```python
from build123d import *

# Parameters (mm, degrees)
ESQUISSE1_W                   = 44.2
ESQUISSE1_H                   = 52.2
BOSS_EXTRU_1_DEPTH            = 52.2
ENL_V_MAT_EXTRU_2_DEPTH       = 74.209903702
ENL_V_MAT_EXTRU_2_DEPTH_BACK  = 44.2
ENL_V_MAT_EXTRU_3_DEPTH       = 74.209903702
ENL_V_MAT_EXTRU_3_DEPTH_BACK  = 44.2
ENL_V_MAT_EXTRU_4_DEPTH       = 78.059003368
ENL_V_MAT_EXTRU_4_DEPTH_BACK  = 46
ENL_V_MAT_EXTRU_5_DEPTH       = 78.059003368
ENL_V_MAT_EXTRU_5_DEPTH_BACK  = 46
ENL_V_MAT_EXTRU_7_DEPTH       = 45.550224466
ENL_V_MAT_EXTRU_7_DEPTH_BACK  = 45.550224466
ENL_V_MAT_EXTRU_8_DEPTH       = 78.059003368
ENL_V_MAT_EXTRU_8_DEPTH_BACK  = 46
ENL_V_MAT_EXTRU_9_DEPTH       = 75.993733072
ENL_V_MAT_EXTRU_9_DEPTH_BACK  = 46
ESQUISSE13_W                  = 35
ESQUISSE13_H                  = 43
ENL_V_MAT_EXTRU_10_DEPTH      = 44
ENL_V_MAT_EXTRU_11_DEPTH      = 72.032809321
ENL_V_MAT_EXTRU_11_DEPTH_BACK = 1.5
ENL_V_MAT_EXTRU_13_DEPTH      = 72.032809321
ENL_V_MAT_EXTRU_13_DEPTH_BACK = 38
ENL_V_MAT_EXTRU_15_DEPTH      = 71.818217995
ENL_V_MAT_EXTRU_15_DEPTH_BACK = 46


with BuildPart() as part:
    # Esquisse1 → Boss.-Extru.1 (new body)
    with BuildSketch(Plane.XY):
        Rectangle(ESQUISSE1_W, ESQUISSE1_H)
    extrude(amount=BOSS_EXTRU_1_DEPTH)

    # Esquisse2 → Enlèv. mat.-Extru.2 (cut, two sides: drawn at the far end of the back side and taken through both)
    with BuildSketch(Plane(origin=(22.1, 0, 0), x_dir=(0, 0, -1), z_dir=(1, 0, 0)).offset(-ENL_V_MAT_EXTRU_2_DEPTH_BACK)):
        Polygon((-201.352290675, -19.9), (-52.2, -19.9), (-28.55, -19.9), (-28.55, -21.45), (-32.25, -21.45), (-32.25, -22.45), (-28.745559959, -26.1), (74.553898465, -133.690091099), (-39.180744024, -409.461834307), (-315.086933163, -295.671743208), align=None)
    extrude(amount=ENL_V_MAT_EXTRU_2_DEPTH + ENL_V_MAT_EXTRU_2_DEPTH_BACK, mode=Mode.SUBTRACT)

    # Esquisse3 → Enlèv. mat.-Extru.3 (cut, two sides: drawn at the far end of the back side and taken through both)
    with BuildSketch(Plane(origin=(22.1, 0, 0), x_dir=(0, 0, -1), z_dir=(1, 0, 0)).offset(-ENL_V_MAT_EXTRU_3_DEPTH_BACK)):
        Polygon((149.152290675, -19.9), (0, -19.9), (-23.65, -19.9), (-23.65, -21.45), (-19.95, -21.45), (-19.95, -22.45), (-23.454440041, -26.1), (-126.753898465, -133.690091099), (-13.019255976, -409.461834307), (262.886933163, -295.671743208), align=None)
    extrude(amount=ENL_V_MAT_EXTRU_3_DEPTH + ENL_V_MAT_EXTRU_3_DEPTH_BACK, mode=Mode.SUBTRACT)

    # Esquisse4 → Enlèv. mat.-Extru.4 (cut, two sides: drawn at the far end of the back side and taken through both)
    with BuildSketch(Plane(origin=(0, 26.1, 0), x_dir=(1, 0, 0), z_dir=(0, 1, 0)).offset(-ENL_V_MAT_EXTRU_4_DEPTH_BACK)):
        Polygon((-15.9, -191.333109619), (-15.9, -52.2), (-15.9, -28.55), (-17.45, -28.55), (-17.45, -32.25), (-18.45, -32.25), (-22.1, -28.745559959), (-122.462816227, 67.614843274), (-379.791464965, -38.281593439), (-273.228648738, -297.229546332), align=None)
    extrude(amount=ENL_V_MAT_EXTRU_4_DEPTH + ENL_V_MAT_EXTRU_4_DEPTH_BACK, mode=Mode.SUBTRACT)

    # Esquisse5 → Enlèv. mat.-Extru.5 (cut, two sides: drawn at the far end of the back side and taken through both)
    with BuildSketch(Plane(origin=(0, 26.1, 0), x_dir=(1, 0, 0), z_dir=(0, 1, 0)).offset(-ENL_V_MAT_EXTRU_5_DEPTH_BACK)):
        Polygon((-15.9, 139.133109619), (-15.9, 0), (-15.9, -23.65), (-17.45, -23.65), (-17.45, -19.95), (-18.45, -19.95), (-22.1, -23.454440041), (-122.462816228, -119.814843274), (-379.791464965, -13.918406561), (-273.228648738, 245.029546332), align=None)
    extrude(amount=ENL_V_MAT_EXTRU_5_DEPTH + ENL_V_MAT_EXTRU_5_DEPTH_BACK, mode=Mode.SUBTRACT)

    # Esquisse6 → Enlèv. mat.-Extru.7 (cut, two sides: drawn at the far end of the back side and taken through both)
    with BuildSketch(Plane.XY.offset(28.55).offset(-ENL_V_MAT_EXTRU_7_DEPTH_BACK)):
        Polygon((-161.22284167, -19.9), (-22.1, -19.9), (-15.9, -19.9), (-15.9, -26.093649616), (-15.9, -165.216491285), (-212.645110561, -361.97019968), (-357.967952231, -216.653708395), align=None)
    extrude(amount=ENL_V_MAT_EXTRU_7_DEPTH + ENL_V_MAT_EXTRU_7_DEPTH_BACK, mode=Mode.SUBTRACT)

    # Esquisse11 → Enlèv. mat.-Extru.8 (cut, two sides: drawn at the far end of the back side and taken through both)
    with BuildSketch(Plane(origin=(0, 26.1, 0), x_dir=(1, 0, 0), z_dir=(0, 1, 0)).offset(-ENL_V_MAT_EXTRU_8_DEPTH_BACK)):
        Polygon((164.227968273, -49.1), (22.1, -49.1), (-15.9, -49.1), (-158.027968273, -49.1), (-158.027968273, -333.355936546), (164.227968273, -333.355936546), align=None)
    extrude(amount=ENL_V_MAT_EXTRU_8_DEPTH + ENL_V_MAT_EXTRU_8_DEPTH_BACK, mode=Mode.SUBTRACT)

    # Esquisse12 → Enlèv. mat.-Extru.9 (cut, two sides: drawn at the far end of the back side and taken through both)
    with BuildSketch(Plane(origin=(0, 26.1, 0), x_dir=(1, 0, 0), z_dir=(0, 1, 0)).offset(-ENL_V_MAT_EXTRU_9_DEPTH_BACK)):
        Polygon((159.687460199, -3.1), (22.1, -3.1), (-15.9, -3.1), (-153.487460199, -3.1), (-153.487460199, 272.074920398), (159.687460199, 272.074920398), align=None)
    extrude(amount=ENL_V_MAT_EXTRU_9_DEPTH + ENL_V_MAT_EXTRU_9_DEPTH_BACK, mode=Mode.SUBTRACT)

    # Esquisse13 → Enlèv. mat.-Extru.10 (cut)
    with BuildSketch(Plane(origin=(0, 26.1, 0), x_dir=(1, 0, 0), z_dir=(0, 1, 0))):
        with Locations((3.1, -26.1)):
            Rectangle(ESQUISSE13_W, ESQUISSE13_H)
    extrude(amount=-ENL_V_MAT_EXTRU_10_DEPTH, mode=Mode.SUBTRACT)

    # Esquisse14 → Enlèv. mat.-Extru.11 (cut, two sides: drawn at the far end of the back side and taken through both)
    with BuildSketch(Plane(origin=(22.1, 0, 0), x_dir=(0, 0, -1), z_dir=(1, 0, 0)).offset(-ENL_V_MAT_EXTRU_11_DEPTH_BACK)):
        with BuildLine():
            Line((-21.6, 4.6), (-21.6, 26.1))
            Line((-21.6, 26.1), (-30.6, 26.1))
            Line((-30.6, 26.1), (-30.6, 4.6))
            ThreePointArc((-30.6, 4.6), (-26.1, 0.1), (-21.6, 4.6))
        make_face()
    extrude(amount=ENL_V_MAT_EXTRU_11_DEPTH + ENL_V_MAT_EXTRU_11_DEPTH_BACK, mode=Mode.SUBTRACT)

    # Esquisse15 → Enlèv. mat.-Extru.13 (cut, two sides: drawn at the far end of the back side and taken through both)
    with BuildSketch(Plane(origin=(22.1, 0, 0), x_dir=(0, 0, -1), z_dir=(1, 0, 0)).offset(-ENL_V_MAT_EXTRU_13_DEPTH_BACK)):
        Polygon((-143.691856556, -19.9), (-28.55, -19.9), (-23.65, -19.9), (91.491856556, -19.9), (91.491856556, -250.183713112), (-143.691856556, -250.183713112), align=None)
    extrude(amount=ENL_V_MAT_EXTRU_13_DEPTH + ENL_V_MAT_EXTRU_13_DEPTH_BACK, mode=Mode.SUBTRACT)

    # Esquisse16 → Enlèv. mat.-Extru.15 (cut, two sides: drawn at the far end of the back side and taken through both)
    with BuildSketch(Plane(origin=(0, -19.9, 0), x_dir=(-1, 0, 0), z_dir=(0, -1, 0)).offset(-ENL_V_MAT_EXTRU_15_DEPTH_BACK)):
        Polygon((15.9, -130.020268394), (15.9, -28.55), (15.9, -23.65), (15.9, 77.820268394), (218.840536787, 77.820268394), (218.840536787, -130.020268394), align=None)
    extrude(amount=ENL_V_MAT_EXTRU_15_DEPTH + ENL_V_MAT_EXTRU_15_DEPTH_BACK, mode=Mode.SUBTRACT)


solid = part.part
```
CAD build for the part. Positions are in the model's coordinates, mm. A direction names the side the tool comes from. Round coordinates to 2 decimals unless told otherwise and drop trailing zeros. Order: outer loops, then holes, each group sorted by start corner. A loop starts at its lowest first (then second) coordinate and runs counter-clockwise, first axis right, second up. Notation, with made-up numbers: (4, 52.5) - (41, 52.5) arc R20 ccw to (41, 70.5) - close; hole circle Ø6 at (-35.5, 12.5). An arc over 180 degrees is marked (long way). Use CSV: the item, a comma, the result in double quotes. Start each with the question number.
1) Saw through at C-C (y = 19.5). List the corners of the cut face in (x, z), and give its area (4 significant figures).
2) Two-plate mould, pull along Z, no slides. Class faces 1 (the flat face through (3, -19.9, 26)), 2 (the flat face through (21, 16, 30.6)), 3 (the flat face through (3, 3, 3.1)): pulls with the +Z half, pulls with the -Z half, needs draft (parallel to the pull), parting line crosses it, or undercut.
3) Saw through at D-D (x = -4). List the corners of the cut face in (y, z).
4) Wall check: L1, parallel to X at y = -3, z = 28; L2, parallel to Z at x = 14, y = 7; L3, parallel to Y at x = 18.5, z = 37. Give the ranges that are in metal, low to high. Write a range as [from, to].
5) Saw through at B-B (z = 26.1). List the corners of the cut face in (x, y).
6) Saw through at A-A (y = -10). List the corners of the cut face in (x, z).
7) Tool access for faces 4 (the flat face through (3, -17.9, 26)), 5 (the flat face through (3, 3, 49.1)), 6 (the cylindrical face through (21.3, 0.1, 26.2)): list every direction of +Z, -Z, +X, -X, +Y, -Y with a clear straight run to the whole face (end or side of a thin tool).
8) Pin check, flat tip, straight feed: pin 1 Ø17.5 at (x, z) = (-4.5, 28) entering from +Y. Stop position of the tip, or through.
Values follow:
1,outline,"(-15.9, 3.1) - (22.1, 3.1) - (22.1, 21.6) - (20.6, 21.6) - (20.6, 4.6) - (-14.4, 4.6) - (-14.4, 47.6) - (20.6, 47.6) - (20.6, 30.6) - (22.1, 30.6) - (22.1, 49.1) - (-15.9, 49.1) - close"
1,area,"229.5 mm2"
2,face 1,"needs draft"
2,face 2,"undercut"
2,face 3,"pulls with the -Z half"
3,outline,"(-19.9, 3.1) - (26.1, 3.1) - (26.1, 4.6) - (-17.9, 4.6) - (-17.9, 47.6) - (26.1, 47.6) - (26.1, 49.1) - (-19.9, 49.1) - close"
4,L1,"x = [-15.9, -14.4], [20.6, 22.1]"
4,L2,"z = [3.1, 4.6], [47.6, 49.1]"
4,L3,"y = [-19.9, -17.9]"
5,outline,"(-15.9, -19.9) - (22.1, -19.9) - (22.1, 0.1) - (20.6, 0.1) - (20.6, -17.9) - (-14.4, -17.9) - (-14.4, 26.1) - (-15.9, 26.1) - close"
6,outline,"(-15.9, 3.1) - (22.1, 3.1) - (22.1, 49.1) - (-15.9, 49.1) - close; hole (-14.4, 4.6) - (20.6, 4.6) - (20.6, 47.6) - (-14.4, 47.6) - close"
7,face 4,"+Y"
7,face 5,"+Z, +X, -X, +Y, -Y"
7,face 6,"+X, +Y"
8,pin 1,"stops at y = -17.9"
